Check sheet for the drawn part. Datum: minimum x, y, z corner. Units: mm. Give positions to 0.01 mm unless a question says otherwise; leave off trailing zeros. Order: outer loops, then holes, each group sorted by start corner. A loop starts at its lowest first (then second) coordinate and runs counter-clockwise, first axis right, second up.
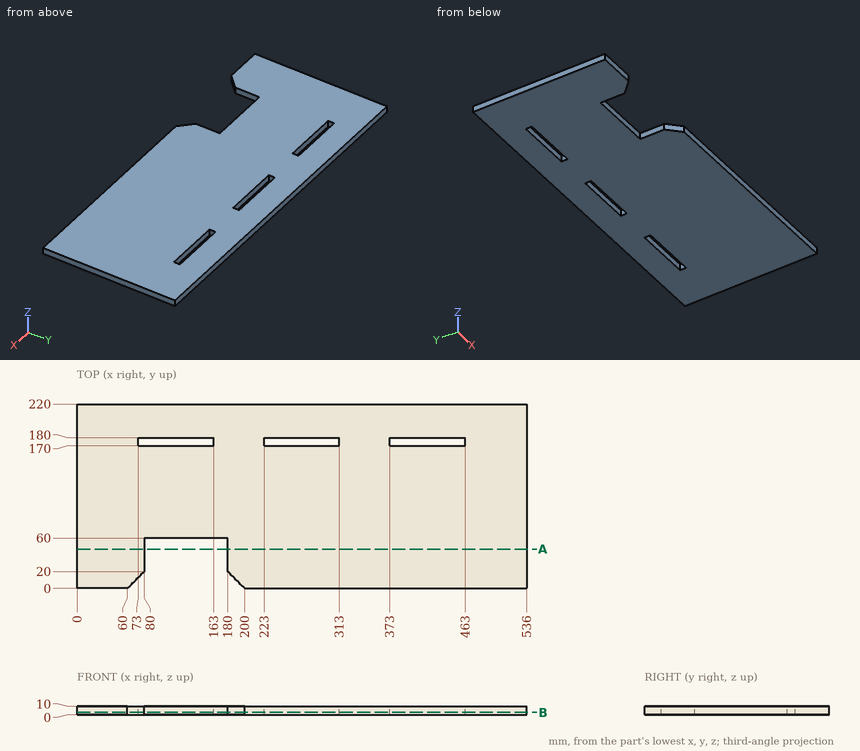
Item 1: Sectioned sample at A-A (y = 47). Enter the section's corners in (x, z).
Reported:
outline: (0, 0) - (80, 0) - (80, 10) - (0, 10) - close; (180, 0) - (536, 0) - (536, 10) - (180, 10) - close
Item 2: Sectioned sample at B-B (z = 3). Enter the section's corners in (x, y).
Reported:
outline: (0, 0) - (60, 0) - (80, 20) - (80, 60) - (180, 60) - (180, 20) - (200, 0) - (536, 0) - (536, 220) - (0, 220) - close; hole (73, 170) - (163, 170) - (163, 180) - (73, 180) - close; hole (223, 170) - (313, 170) - (313, 180) - (223, 180) - close; hole (373, 170) - (463, 170) - (463, 180) - (373, 180) - close
Item 3: Scan lines: L1, parallel to X at y = 177.5, z = 7.75; L2, parallel to X at y = 31.5, z = 0.75; L3, parallel to Y at x = 394.5, z = 5.25. Record each from-to range of solid material in increasing order.
Reported:
L1: x = 0 to 73, 163 to 223, 313 to 373, 463 to 536
L2: x = 0 to 80, 180 to 536
L3: y = 0 to 170, 180 to 220
Item 4: Gauge pin test, flat end, axial feed: pin 1 (5 mm diameter, centred on x = 105.5, z = 3, fed in from -Y). Record the tip position at first contact, or that the pin passes through.
Reported:
pin 1: stops at y = 60
